Geometry check sheet. Reference: the model listing, model coordinates, mm. Face numbers are marked on the shaded views. A direction names the side the tool comes from. Coordinates: 2 decimals unless noted, no trailing zeros. Loops run counter-clockwise (first coordinate to the right, second up) from the corner with the lowest first, then second, coordinate; pieces in that order, holes last.
from build123d import *

# Parameters (mm, degrees)
SKETCH1_R           = 1.5
BOSS_EXTRUDE1_DEPTH = 8.4


with BuildPart() as part:
    # Sketch1 → Boss-Extrude1 (new body)
    with BuildSketch(Plane(origin=(0, 0, 0), x_dir=(1, 0, 0), z_dir=(0, 1, 0))):
        with BuildLine():
            Line((-28.3, 11), (-22.3, 11))
            Line((-22.3, 11), (-22.3, 8))
            Line((-22.3, 8), (-23.8, 8))
            Line((-23.8, 8), (-23.8, 5))
            Line((-23.8, 5), (-22.3, 5))
            Line((-22.3, 5), (-22.3, 4))
            Line((-22.3, 4), (-18.3, 4))
            Line((-18.3, 4), (-18.3, 5))
            Line((-18.3, 5), (-16.8, 5))
            Line((-16.8, 5), (-16.8, 8))
            Line((-16.8, 8), (-18.3, 8))
            Line((-18.3, 8), (-18.3, 11))
            Line((-18.3, 11), (-14.3, 11))
            Line((-14.3, 11), (-14.3, 19))
            Line((-14.3, 19), (-6.7, 19))
            Line((-6.7, 19), (-6.7, 11))
            Line((-6.7, 11), (2.3, 11))
            Line((2.3, 11), (2.3, 19))
            Line((2.3, 19), (9.9, 19))
            Line((9.9, 19), (9.9, 11))
            Line((9.9, 11), (13.1, 11))
            Line((13.1, 11), (13.1, 8))
            Line((13.1, 8), (11.6, 8))
            Line((11.6, 8), (11.6, 5))
            Line((11.6, 5), (13.1, 5))
            Line((13.1, 5), (13.1, 4))
            Line((13.1, 4), (17.1, 4))
            Line((17.1, 4), (17.1, 5))
            Line((17.1, 5), (18.6, 5))
            Line((18.6, 5), (18.6, 8))
            Line((18.6, 8), (17.1, 8))
            Line((17.1, 8), (17.1, 11))
            Line((17.1, 11), (28.3, 11))
            Line((28.3, 11), (28.3, -11))
            Line((28.3, -11), (19.3, -11))
            ThreePointArc((19.3, -11), (6.8, 1.5), (-5.7, -11))
            Line((-5.7, -11), (-28.3, -11))
            Line((-28.3, -11), (-28.3, 11))
        make_face()
        with Locations((-8.7, 0)):
            Circle(SKETCH1_R, mode=Mode.SUBTRACT)
        with Locations((22.3, 0)):
            Circle(SKETCH1_R, mode=Mode.SUBTRACT)
    extrude(amount=BOSS_EXTRUDE1_DEPTH)


solid = part.part
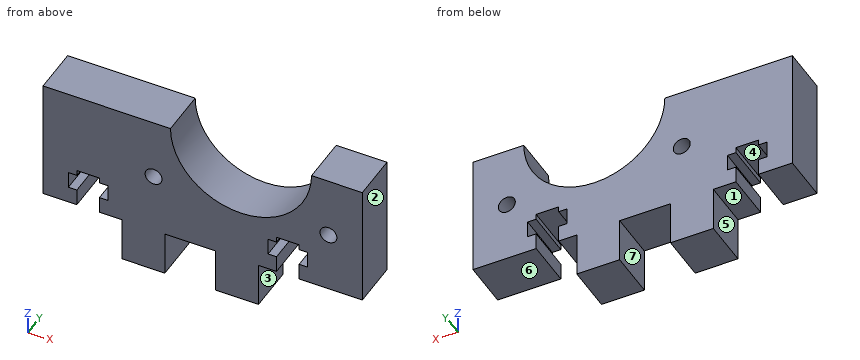
1) Section check C-C on y = 3. Count the separate pieces of the cut face and the enclosed holes in it, and give its area (3 significant figures).
Data:
separate pieces: 1
enclosed holes: 2
area: 1,030 mm2
2) Section check B-B on z = 0. Record the cut outline in (x, y), and give its area (3 significant figures).
Data:
outline: (-28.3, 0) - (-10.2, 0) - (-10.2, 8.4) - (-28.3, 8.4) - close; (-7.2, 0) - (0.86, 0) - (0.86, 8.4) - (-7.2, 8.4) - close; (12.74, 0) - (20.8, 0) - (20.8, 8.4) - (12.74, 8.4) - close; (23.8, 0) - (28.3, 0) - (28.3, 8.4) - (23.8, 8.4) - close
area: 325 mm2
3) Mould release check, pull along X, two halves, no side actions. Record for the marked faces 5, 6 and 7: +X half, -X half, draft (parallel to the pull), parting line (faces both ways), or undercut.
Data:
face 5: -X half
face 6: draft
face 7: undercut
4) Section check D-D on x = 22.3. Record the cut outline in (y, z).
Data:
outline: (0, -11) - (8.4, -11) - (8.4, -1.5) - (0, -1.5) - close; (0, 1.5) - (8.4, 1.5) - (8.4, 11) - (0, 11) - close
5) Access from +Z, -Z, +X, -X, +Y, -Y to the whole of each face (thin tool, end or side, straight path). Record for the marked faces 1, 2, 3 and 4.
Data:
face 1: -Z, -X, +Y, -Y
face 2: +Z, -Z, +X, +Y, -Y
face 3: -Z, +X, +Y, -Y
face 4: -Z, +Y, -Y
6) Section check A-A on x = -8.7. Record the cut outline in (y, z).
Data:
outline: (0, -19) - (8.4, -19) - (8.4, -1.5) - (0, -1.5) - close; (0, 1.5) - (8.4, 1.5) - (8.4, 11) - (0, 11) - close
7) Material ranges on probe 1 along X at (y, z) = (1.75, -5.75); probe 2 along X at (y, z) = (7.25, -15.75); probe 3 along Z at (x, y) = (-8.7, 2.5), recorded low to high.
Data:
probe 1: x = -28.3 to -23.8, -16.8 to 11.6, 18.6 to 28.3
probe 2: x = -14.3 to -6.7, 2.3 to 9.9
probe 3: z = -19 to -1.5, 1.5 to 11
8) Depth check by flat-ended pin: pin 1 (0.8 mm diameter, centred on x = 12.5, y = 4, fed in from -Z); pin 2 (1.8 mm diameter, centred on x = -8.7, z = 0, fed in from -Y). Enter the tip coordinate at first touch or a pass-through.
Data:
pin 1: stops at z = -11
pin 2: passes through
